Geometry: see drawing. Coordinates: mm, zero at the bounding-box minimum. A direction names the side the tool comes from. Coordinates: 2 decimals unless noted, no trailing zeros. Write each loop counter-clockwise with the first axis right and the second up, starting at its lowest first coordinate (ties: lowest second). Pieces come first, ordered by that corner, then holes. Notation, with made-up numbers: (32.25, -21) -> (57.25, -21) arc R12 cw to (57.25, -10) -> close; hole circle Ø1 at (7, 82.25). An arc over 180 degrees is marked (long way). Use one line per item in the form item = value. Start each with the question number.
(1) First-contact query: pin 1 (13.5 mm diameter, centred on x = 231, y = 24.5, fed in from -Z); pin 2 (4 mm diameter, centred on y = 41, z = 25.5, fed in from -X); pin 3 (2 mm diameter, centred on y = 30.5, z = 16.5, fed in from -X). Flat tips, straight axial feed; report the tip coordinate or a pass-through.
(2) Set-up query: the marked faces 3, 4, 5 and 6. Return all of +Z, -Z, +X, -X, +Y, -Y with unobstructed straight access to the full face (end or side cutting, diameter ignored); none if empty.
(3) Cut plane A-A on x = 207. Return the cut outline in (y, z) (3 decimals).
(4) Ray query, line 1 along X through (y, z) = (3, 32); line 2 along Z through (x, y) = (415, 23.5) (3 decimals); line 3 along X through (y, z) = (27, 31.5). Return the intervals inside material, ascending.
(5) Pull-direction query (X, two-part tool) for the marked faces 1 and 2; classes: released by +X, released by -X, zero draft, split by the parting line, or undercut.
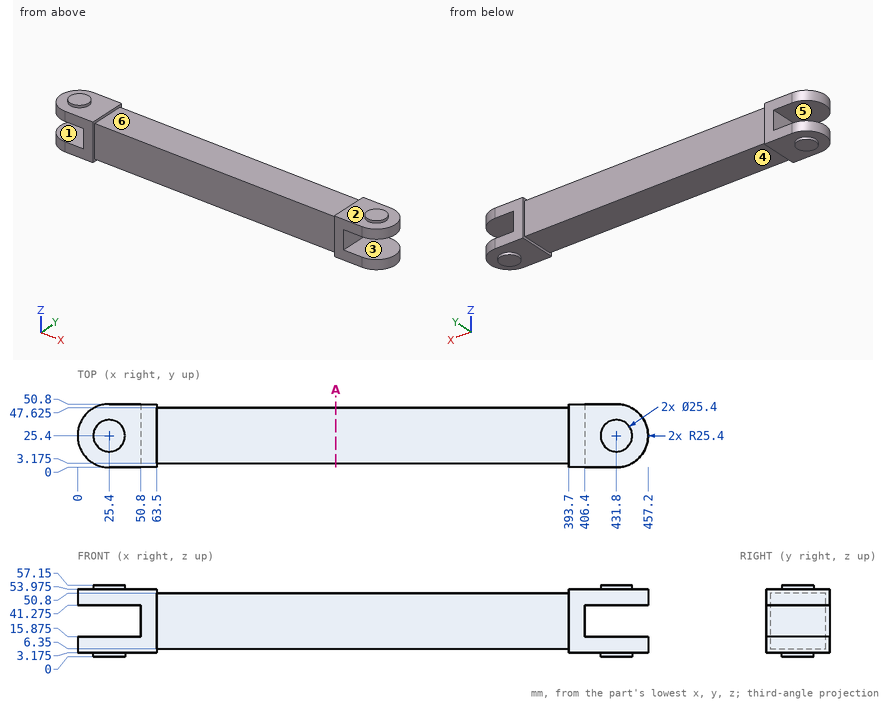
Values:
q1.pin_1 = 6.35
q1.pin_2 = 50.8
q1.pin_3 = 0.37
q2.face_3 = +X, +Y, -Y
q2.face_4 = -Z, +Y, -Y
q2.face_5 = -X, +Y, -Y
q2.face_6 = +Z, +Y, -Y
q3.outline = (3.175, 6.35) -> (47.625, 6.35) -> (47.625, 50.8) -> (3.175, 50.8) -> close
q4.line_1 = 50.8 to 63.5, 393.7 to 406.4
q4.line_2 = 3.175 to 15.875, 41.275 to 53.975
q4.line_3 = 50.8 to 406.4
q5.face_1 = zero draft
q5.face_2 = undercut
